Can you work these out from the drawing? Everything is in mm from the part's minimum corner. A direction names the side the tool comes from. Give positions to 0.01 mm unless a question says otherwise; leave off trailing zeros. Order: outer loops, then holes, each group sorted by start corner. A loop starts at its lowest first (then second) coordinate and runs counter-clockwise, first axis right, second up. Notation, with made-up numbers: (61.25, 62.5) - (114.25, 62.5) arc R34 cw to (114.25, 99.5) - close; hole circle Ø8 at (61, -10.5). An arc over 180 degrees is marked (long way). Write each question's results on one line, items separated by ' | '. Start each with the question number.
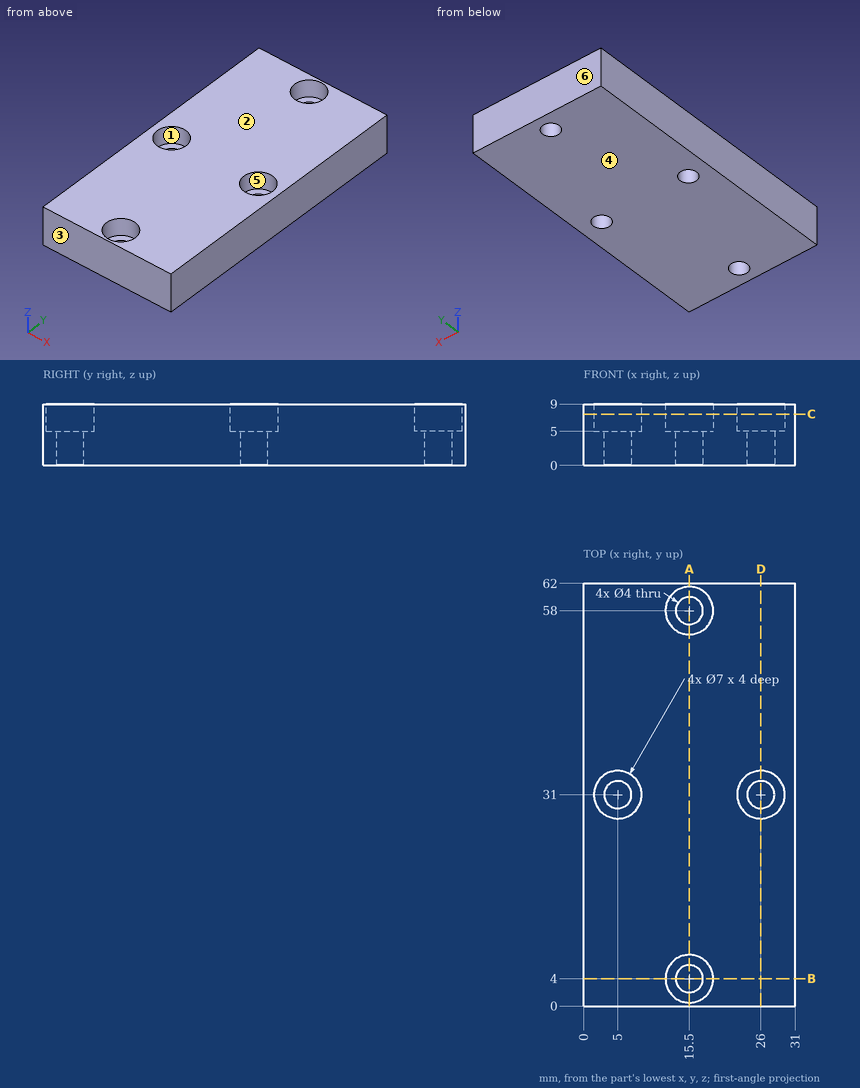
Q1. Will these pins go through, and if not, where does the flat tip stop? P1, Ø7.5, axis at x = 14.5, y = 59, coming from the +Z side; P2, Ø3.5, axis at x = 6.5, y = 30.5, coming from the +Z side.
Q2. If we section it at A-A (x = 15.5): Please give me the cut outline in (y, z), plus the area to 3 significant figures.
Q3. If I drill on probe 1 along Y at (x, z) = (15.5, 7.7); probe 2 along X at (y, z) = (29.5, 3.5); probe 3 along Y at (x, z) = (5, 3.7), over which ranges is the centre line in solid material (lowest first)? Write a range as from..to.
Q4. Thinking about a two-plate mould opening in Y: for the marked faces 3, 4, 5 and 6, which applies, released by +Y, released by -Y, zero draft, split by the parting line, or undercut?
Q5. If we section it at D-D (x = 26): Please give me the cut outline in (y, z), plus the area to 3 significant figures.
Q6. Which directions (+Z, -Z, +X, -X, +Y, -Y) give clear straight access to the entire face, cutting with the end or side of a thin tool? Please do the marked faces 1 and 2.
Q7. If we section it at B-B (y = 4): Please give me the cut outline in (x, z), plus the area to 3 significant figures.
Q8. If we section it at C-C (z = 7.5): Please give me the cut outline in (x, y), plus the area to 3 significant figures.
Findings below:
1) P1: stops at z = 9 | P2: stops at z = 5
2) outline: (0, 0) - (2, 0) - (2, 5) - (0.5, 5) - (0.5, 9) - (0, 9) - close; (6, 0) - (56, 0) - (56, 5) - (54.5, 5) - (54.5, 9) - (7.5, 9) - (7.5, 5) - (6, 5) - close; (60, 0) - (62, 0) - (62, 9) - (61.5, 9) - (61.5, 5) - (60, 5) - close | area: 462 mm2
3) probe 1: y = 0..0.5, 7.5..54.5, 61.5..62 | probe 2: x = 0..3.68, 6.32..24.68, 27.32..31 | probe 3: y = 0..29, 33..62
4) face 3: released by -Y | face 4: zero draft | face 5: undercut | face 6: released by +Y
5) outline: (0, 0) - (29, 0) - (29, 5) - (27.5, 5) - (27.5, 9) - (0, 9) - close; (33, 0) - (62, 0) - (62, 9) - (34.5, 9) - (34.5, 5) - (33, 5) - close | area: 510 mm2
6) face 1: +Z | face 2: +Z, +X, -X, +Y, -Y
7) outline: (0, 0) - (13.5, 0) - (13.5, 5) - (12, 5) - (12, 9) - (0, 9) - close; (17.5, 0) - (31, 0) - (31, 9) - (19, 9) - (19, 5) - (17.5, 5) - close | area: 231 mm2
8) outline: (0, 0) - (31, 0) - (31, 62) - (0, 62) - close; hole circle Ø7 at (5, 31); hole circle Ø7 at (15.5, 4); hole circle Ø7 at (15.5, 58); hole circle Ø7 at (26, 31) | area: 1,770 mm2
